Autodesk Inventor part; units mm, degrees
ref_plane "Work Plane1" through (0, 1.5, 0) normal (0, 1, 0) x (1, 0, 0)
ref_plane "YZ Plane" through (0, 0, 0) normal (1, 0, 0) x (0, 1, 0)
ref_plane "XZ Plane" through (0, 0, 0) normal (0, 1, 0) x (-1, 0, 0)
sketch "Sketch1" plane through (0, 0, 0) normal (0, 1, 0) x (-1, 0, 0)
  circle A0 centre (0, 0) radius 5
  circle A1 centre (-30, 20) radius 5
  line L0 (-4.715, -1.6641) -> (-29.7226, 15.0077)
  line L1 (-0.2774, 4.9923) -> (-25.285, 21.6641)
  line L2 (0, 0) -> (-30, 0) construction
  line L3 (-30, 0) -> (-30, 20) construction
  line L4 (0, 0) -> (-30, 20) construction
  dimension "d0" = 10
  dimension "d1" = 10
  dimension "d2" = 4
  dimension "d3" = 4
  dimension "d4" = 30
  dimension "d5" = 20
extrude "Extrusion1" add sketch "Sketch1" along normal blind 5
sketch "Sketch2" plane through (0, 0, 0) normal (0, -1, 0) x (1, 0, 0)
  line L0 (0, 0) -> (30, 20) construction
  arc A0 (29.7226, 15.0077) -> (25.285, 21.6641) centre (30, 20) ccw
  line L1 (0.2774, 4.9923) -> (25.285, 21.6641)
  arc A1 (0.2774, 4.9923) -> (4.715, -1.6641) centre (0, 0) ccw
  line L2 (29.7226, 15.0077) -> (4.715, -1.6641)
hole "Hole1" at (30, 0, 20) direction (0, 1, 0) diameter 3.1 end through all
ref_plane "Work Plane1" through (0, 1.5, 0) normal (0, 1, 0) x (1, 0, 0)
sketch "Sketch4" plane through (0, 5, 0) normal (0, 1, 0) x (1, 0, 0)
  circle A0 centre (30, -20) radius 1.55
  arc A1 (25.285, -21.6641) -> (29.7226, -15.0077) centre (30, -20) ccw
  line L0 (29.7226, -15.0077) -> (4.715, 1.6641)
  arc A2 (4.715, 1.6641) -> (0.2774, -4.9923) centre (0, 0) ccw
  line L1 (0.2774, -4.9923) -> (25.285, -21.6641)
hole "Hole2" at (0, 5, 0) direction (0, -1, 0) diameter 2.459 end through all
properties part number "gripper_hand_connector"
Verification items for the finished model (mm, model axes). Round coordinates to 2 decimals unless told otherwise and drop trailing zeros. Write each loop counter-clockwise with the first axis right and the second up, starting at its lowest first coordinate (ties: lowest second). Pieces come first, ordered by that corner, then holes. Notation, with made-up numbers: (60, -19) - (114, -19) arc R14 ccw to (114, 6) - close; hole circle Ø11 at (-37, 61.5). An arc over 180 degrees is marked (long way). Answer as a JSON object with one key per item and string values. Group by question number.
Q1. Go/stop test with flat-tipped pins: pin 1 Ø1 at (y, z) = (1, 10) entering from -X; pin 2 Ø3 at (y, z) = (2, 18) entering from +X. Record where each tip stops, or that it passes through.
Q2. Thickness scan on line 1 (Z direction, x = 0, y = 2.9); line 2 (Z direction, x = 30, y = 1.5); line 3 (X direction, y = 2.8, z = 0). Record the ranges inside material, lowest first.
Q3. Section check A-A, the plane z = -0.5. Enter the section's corners in (x, y).
Q4. Section check D-D, the plane x = 4. Enter the section's corners in (y, z), plus the area to 3 significant figures.
Q5. Section check C-C, the plane z = 20. Enter the section's corners in (x, y), plus the area to 3 significant figures.
Q6. Section check B-B, the plane y = 1.8. Give the number of separate pieces and of enclosed holes in the cut face, plus the area to 3 significant figures.
Q7. Mould release check, pull along Z, two halves, no side actions. Record for faces 1 (the flat face through (12.606, 2.465, 13.211)), 2 (the cylindrical face through (0.748, 2.465, -0.976)), 3 (the cylindrical face through (34, 2, 23)): released by +Z, released by -Z, zero draft, split by the parting line, or undercut.
Found:
{
 "1": {"pin 1": "stops at x = 7.04", "pin 2": "stops at x = 34.97"},
 "2": {"line 1": "z = -5 to -1.23, 1.23 to 5", "line 2": "z = 15 to 18.45, 21.55 to 25", "line 3": "x = -5 to -1.23, 1.23 to 7.21"},
 "3": {"outline": "(-4.97, 0) - (-1.12, 0) - (-1.12, 5) - (-4.97, 5) - close; (1.12, 0) - (6.46, 0) - (6.46, 5) - (1.12, 5) - close"},
 "4": {"outline": "(0, -3) - (5, -3) - (5, 7.47) - (0, 7.47) - close", "area": "52.4 mm^2"},
 "5": {"outline": "(22.79, 0) - (28.45, 0) - (28.45, 5) - (22.79, 5) - close; (31.55, 0) - (35, 0) - (35, 5) - (31.55, 5) - close", "area": "45.6 mm^2"},
 "6": {"separate pieces": "1", "enclosed holes": "2", "area": "363 mm^2"},
 "7": {"face 1": "released by +Z", "face 2": "undercut", "face 3": "split by the parting line"}
}
